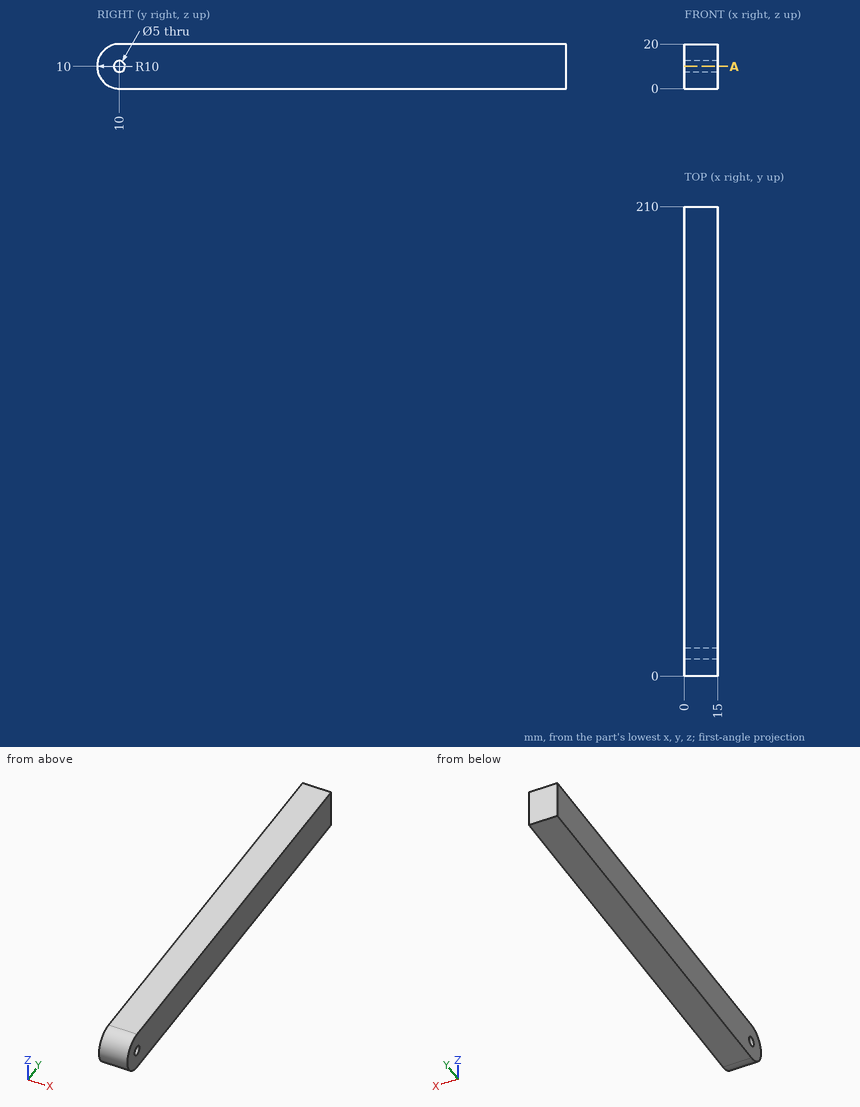
Print and shaded views of the part. All mm, measured from the part's lowest x, y and z. Coordinates: 2 decimals unless noted, no trailing zeros. Loops run counter-clockwise (first coordinate to the right, second up) from the corner with the lowest first, then second, coordinate; pieces in that order, holes last. Notation, with made-up numbers: (55, 10) -> (90, 10) arc R20 cw to (90, 39) -> close; hole circle Ø6 at (23.5, -11). An arc over 180 degrees is marked (long way). Use one line per item in the form item = value. Start each with the question number.
(1) Probe probe 1 along Y at (x, z) = (3.75, 10); probe 2 along Z at (x, y) = (2.75, 11); probe 3 along Y at (x, z) = (8.5, 8). List the from-to ranges inside material, lowest first. Write a range as from..to.
(2) Flat gauge pin, fed straight in: pin 1 (2 mm diameter, centred on x = 10, z = 5, fed in from -Y). Where does the tip first touch, or does it go through?
(3) Cut at A-A on z = 10. Give the cut face in (x, y), and give its area (4 significant figures).
Values:
q1.probe_1 = 0..7.5, 12.5..210
q1.probe_2 = 0..7.71, 12.29..20
q1.probe_3 = 0.2..8.5, 11.5..210
q2.pin_1 = 0.83
q3.outline = (0, 0) -> (15, 0) -> (15, 7.5) -> (0, 7.5) -> close; (0, 12.5) -> (15, 12.5) -> (15, 210) -> (0, 210) -> close
q3.area = 3,075 mm2
